Autodesk Inventor part; units mm, degrees
ref_plane "YZ Plane" through (0, 0, 0) normal (1, 0, 0) x (0, 1, 0)
ref_plane "XZ Plane" through (0, 0, 0) normal (0, 1, 0) x (-1, 0, 0)
ref_plane "XY Plane" through (0, 0, 0) normal (0, 0, 1) x (1, 0, 0)
sketch "Sketch1" plane through (0, 0, 0) normal (0, 0, 1) x (1, 0, 0)
  circle A0 centre (0, 0) radius 3.75
  dimension "d0" = 7.5
extrude "Extrusion1" add sketch "Sketch1" along normal blind 21
sketch "Sketch2" plane through (0, 0, 21) normal (0, 0, 1) x (1, 0, 0)
  circle A0 centre (0, 0) radius 3.75
  line L0 (-2.7951, 2.5) -> (2.7951, 2.5)
  dimension "d3" = 2.5
extrude "Extrusion2" cut sketch "Sketch2" against normal through all contours L0 A0 picked at (-0.7066, 2.6978)
sketch "Sketch3" plane through (0, 0, 0) normal (0, 0, -1) x (-1, 0, 0)
  circle A0 centre (0, 0) radius 4
  dimension "d6" = 8
extrude "Extrusion3" add sketch "Sketch3" against normal blind 1
properties material "Stainless Steel"
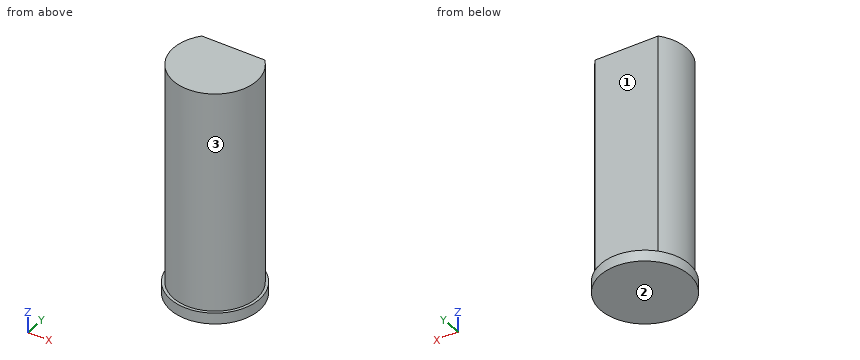
Model file for the job. Use its own axes, mm. Face numbers are marked on the shaded views. A direction names the side the tool comes from. Round coordinates to 2 decimals unless told otherwise and drop trailing zeros. Order: outer loops, then holes, each group sorted by start corner. A loop starts at its lowest first (then second) coordinate and runs counter-clockwise, first axis right, second up.
(1) Band-saw the part on D-D (y = 2.75). List the corners of the cut face in (x, z).
(2) Drill centre lines: line 1 (X direction, y = -2.5, z = 17); line 2 (X direction, y = 0, z = 6.75); line 3 (Y direction, x = -2.5, z = 7). Where is each one in solid material? Low to high.
(3) Band-saw the part on C-C (z = 8). List the corners of the cut face in (x, y).
(4) Band-saw the part on B-B (y = 0). List the corners of the cut face in (x, z), then the cut area to 3 significant figures.
(5) 3-axis set-ups, long thin cutter, end or side, ignore diameter. For the marked faces 1, 2 and 3: which of +Z, -Z, +X, -X, +Y, -Y reach the whole face in a straight line?
(6) Band-saw the part on A-A (x = 0). List the corners of the cut face in (y, z), then the cut area to 3 significant figures.
(7) Pin check, flat tips, straight feed: pin 1 (1 mm diameter, centred on y = -1.5, z = 13.5, fed in from -X); pin 2 (4 mm diameter, centred on x = 2.5, z = 17, fed in from -Y); pin 3 (4.5 mm diameter, centred on x = 1.5, z = 9, fed in from +Y). Stop position of each tip, or through.
Verdict:
1. outline: (-2.9, 0) - (2.9, 0) - (2.9, 1) - (-2.9, 1) - close
2. line 1: x = -2.8 to 2.8
2. line 2: x = -3.75 to 3.75
2. line 3: y = -2.8 to 2.5
3. outline: (-2.8, 2.5) arc R3.75 ccw (long way) to (2.8, 2.5) - close
4. outline: (-4, 0) - (4, 0) - (4, 1) - (3.75, 1) - (3.75, 21) - (-3.75, 21) - (-3.75, 1) - (-4, 1) - close
4. area: 158 mm2
5. face 1: +Z, +X, -X, +Y
5. face 2: -Z, +X, -X, +Y, -Y
5. face 3: +Z
6. outline: (-4, 0) - (4, 0) - (4, 1) - (2.5, 1) - (2.5, 21) - (-3.75, 21) - (-3.75, 1) - (-4, 1) - close
6. area: 133 mm2
7. pin 1: stops at x = -3.61
7. pin 2: stops at y = -3.72
7. pin 3: stops at y = 2.5
